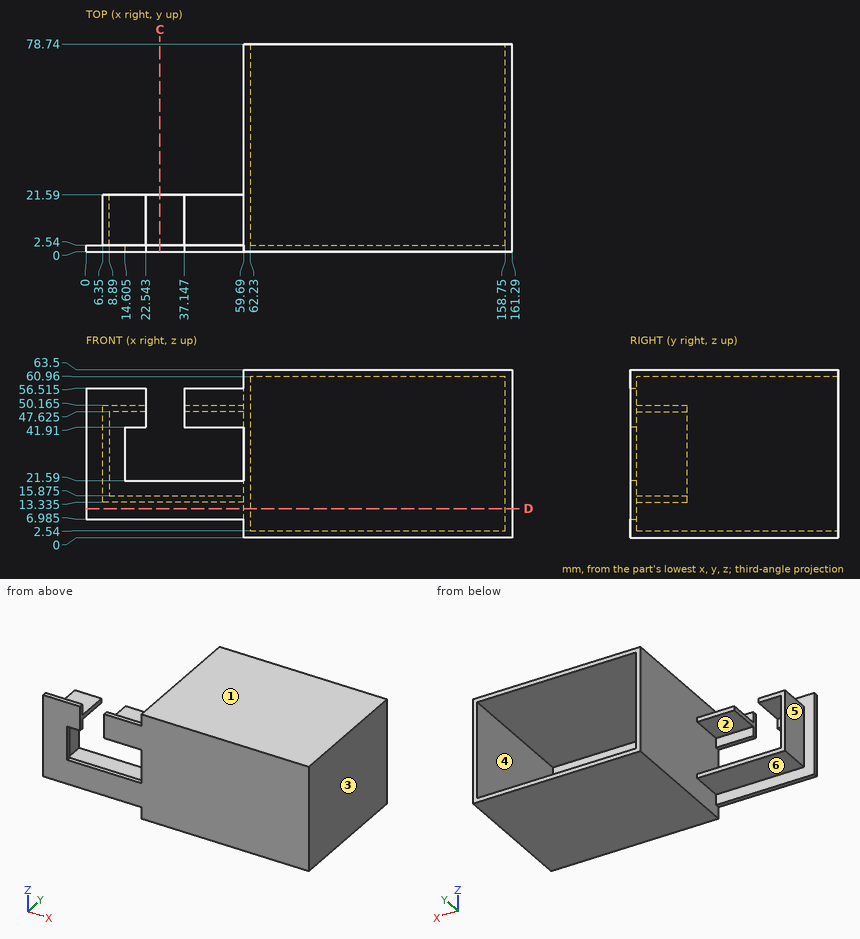
Job drawing, mm, ordinate dimensions from the low corner. One solid piece. A direction names the side the tool comes from. Coordinates: 2 decimals unless noted, no trailing zeros. Order: outer loops, then holes, each group sorted by start corner. A loop starts at its lowest first (then second) coordinate and runs counter-clockwise, first axis right, second up. Notation, with made-up numbers: (21, -9) -> (36, -9) arc R31 cw to (36, 15) -> close; hole circle Ø1 at (40.5, 10.5). An arc over 180 degrees is marked (long way). Put each result on its own line as item: value. Start each with the question number.
(1) Probe line 1 along X through (y, z) = (5, 18); line 2 along X through (y, z) = (69.5, 43); line 3 along Z through (x, y) = (116, 31). List the from-to ranges inside material, lowest first. Write a range as [from, to].
(2) Mould opens along Z. For the marked faces 1, 2 and 3 say: pulls with the +Z half, pulls with the -Z half, needs draft (parallel to the pull), parting line crosses it, or undercut.
(3) Pin check, flat tips, straight feed: pin 1 Ø0.8 at (x, y) = (48.5, 1) entering from +Z (1 decimal); pin 2 Ø1.5 at (x, z) = (88, 54) entering from +Y; pin 3 Ø19 at (y, z) = (25.5, 27.5) entering from -X. Stop position of each tip, or through.
(4) Band-saw the part on C-C (x = 28). Give the cut face in (y, z) (1 decimal).
(5) Which spindle directions (+Z, -Z, +X, -X, +Y, -Y) get a long thin tool onto all of the face, cutting with end or side? Do the marked faces 4, 5 and 6. Say none if no direction does.
(6) Band-saw the part on D-D (z = 11). Give the cut face in (x, y).
Determined:
1. line 1: x = [6.35, 8.89], [59.69, 62.23], [158.75, 161.29]
1. line 2: x = [59.69, 62.23], [158.75, 161.29]
1. line 3: z = [0, 2.54], [60.96, 63.5]
2. face 1: pulls with the +Z half
2. face 2: undercut
2. face 3: needs draft
3. pin 1: stops at z = 56.5
3. pin 2: stops at y = 2.54
3. pin 3: stops at x = 6.35
4. outline: (0, 7) -> (2.5, 7) -> (2.5, 13.3) -> (21.6, 13.3) -> (21.6, 15.9) -> (2.5, 15.9) -> (2.5, 21.6) -> (0, 21.6) -> close
5. face 4: +Y
5. face 5: +Z, -Z, -X, +Y
5. face 6: -Z, -X, +Y
6. outline: (0, 0) -> (161.29, 0) -> (161.29, 78.74) -> (158.75, 78.74) -> (158.75, 2.54) -> (62.23, 2.54) -> (62.23, 78.74) -> (59.69, 78.74) -> (59.69, 2.54) -> (0, 2.54) -> close
